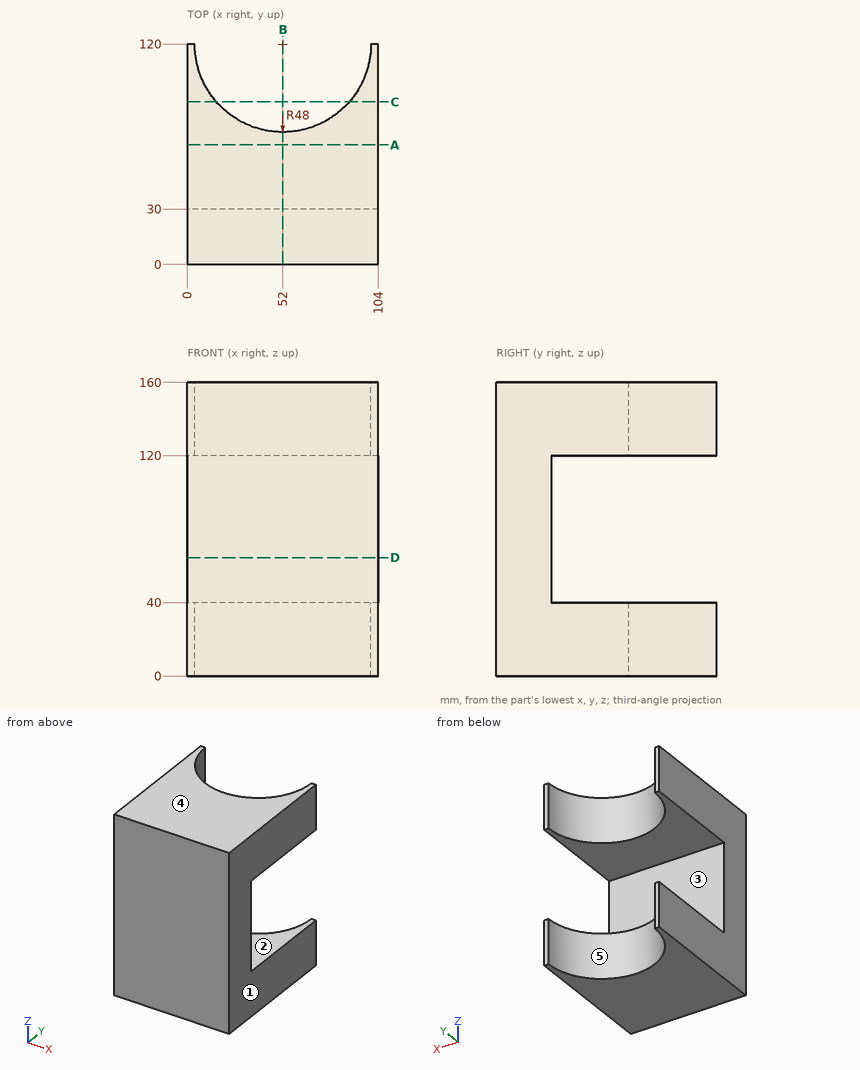
Geometry: see drawing. Coordinates: mm, zero at the bounding-box minimum. A direction names the side the tool comes from. Give positions to 0.01 mm unless a question says otherwise; leave off trailing zeros. Write each loop counter-clockwise with the first axis right and the second up, starting at its lowest first coordinate (ties: lowest second). Pieces come first, ordered by that corner, then holes. Notation, with made-up numbers: (-11.5, -10) -> (13.5, -10) arc R21 ccw to (13.5, 1) -> close; hole circle Ø2 at (9, 73.25). An arc over 180 degrees is marked (long way). Use one line per item in the form item = value. Start each with the question number.
1) Set-up query: the marked faces 1 and 2. Return all of +Z, -Z, +X, -X, +Y, -Y with unobstructed straight access to the full face (end or side cutting, diameter ignored); none if empty.
2) Section query C-C on y = 88.5. Return the cut outline in (x, z), then the cut area to 3 significant figures.
3) Section query B-B on x = 52. Return the cut outline in (y, z), then the cut area to 3 significant figures.
4) Pin query (flat end, axial travel): pin 1 (3 mm diameter, centred on x = 24, z = 97, fed in from +Y); pin 2 (12 mm diameter, centred on x = 87, z = 30, fed in from +Y). Return the tip coordinate at first contact, or that it passes through.
5) Section query D-D on z = 64.5. Return the cut outline in (x, y), then the cut area to 3 significant figures.
6) Section query A-A on y = 65. Return the cut outline in (x, z), then the cut area to 3 significant figures.
7) Ray query, probe 1 along Z at (x, y) = (47, 47); probe 2 along Y at (x, z) = (6, 88); probe 3 along X at (y, z) = (96, 35.5). Return the intervals inside material, ascending. Write a range as from..to.
8) Draft query along Z for the marked faces 3, 4 and 5. Return one class per face: pulls with the +Z half, pulls with the -Z half, needs draft (parallel to the pull), parting line crosses it, or undercut.
Outcome:
q1.face_1 = +Z, -Z, +X, +Y, -Y
q1.face_2 = +X, -X, +Y
q2.outline = (0, 0) -> (15.78, 0) -> (15.78, 40) -> (0, 40) -> close; (0, 120) -> (15.78, 120) -> (15.78, 160) -> (0, 160) -> close; (88.22, 0) -> (104, 0) -> (104, 40) -> (88.22, 40) -> close; (88.22, 120) -> (104, 120) -> (104, 160) -> (88.22, 160) -> close
q2.area = 2,530 mm^2
q3.outline = (0, 0) -> (72, 0) -> (72, 40) -> (30, 40) -> (30, 120) -> (72, 120) -> (72, 160) -> (0, 160) -> close
q3.area = 8,160 mm^2
q4.pin_1 = 30
q4.pin_2 = 95.04
q5.outline = (0, 0) -> (104, 0) -> (104, 30) -> (0, 30) -> close
q5.area = 3,120 mm^2
q6.outline = (0, 0) -> (104, 0) -> (104, 40) -> (0, 40) -> close; (0, 120) -> (104, 120) -> (104, 160) -> (0, 160) -> close
q6.area = 8,320 mm^2
q7.probe_1 = 0..40, 120..160
q7.probe_2 = 0..30
q7.probe_3 = 0..10.43, 93.57..104
q8.face_3 = undercut
q8.face_4 = pulls with the +Z half
q8.face_5 = needs draft
